Autodesk Inventor part; units mm, degrees
ref_plane "YZ Plane" through (0, 0, 0) normal (1, 0, 0) x (0, 1, 0)
ref_plane "XZ Plane" through (0, 0, 0) normal (0, 1, 0) x (-1, 0, 0)
ref_plane "XY Plane" through (0, 0, 0) normal (0, 0, 1) x (1, 0, 0)
sketch "Sketch1" plane through (0, 0, 0) normal (0, 0, 1) x (1, 0, 0)
  circle A0 centre (0, 0) radius 13.75
  circle A1 centre (0, 0) radius 18.75
  line L0 (-18.75, 0) -> (-38, 0)
  line L1 (-38, 0) -> (-38, -5)
  line L2 (-38, -5) -> (-18.75, -5)
  line L3 (-18.75, -5) -> (-18.75, 0)
  line L4 (-18.75, -5) -> (-13.75, -5)
  line L5 (-13.75, -5) -> (-13.75, 0)
  line L6 (-13.75, 0) -> (-18.75, 0)
  line L7 (-18.75, 0) -> (-18.75, -5)
  line L8 (18.75, 0) -> (38, 0)
  line L9 (38, 0) -> (38, -5)
  line L10 (38, -5) -> (18.75, -5)
  line L11 (18.75, -5) -> (18.75, 0)
  line L12 (18.75, -5) -> (13.75, -5)
  line L13 (13.75, -5) -> (13.75, 0)
  line L14 (13.75, 0) -> (18.75, 0)
  line L15 (18.75, 0) -> (18.75, -5)
  point P0 (-18.071, -5)
  point P1 (18.071, -5)
  dimension "d0" = 27.5
  dimension "d1" = 5
  dimension "d2" = 5
  dimension "d3" = 19.25
  dimension "d4" = 19.25
  dimension "d5" = 5
extrude "Extrusion1" add sketch "Sketch1" along normal blind 10 contours L13 L12 A1 L4 L5 A0 | L14 A1 L12 L13 | L5 L4 A1 L6 | L11 L12 A1 | L8 L9 L10 L11 | L3 L2 L1 L0 | A1 L4 L3
sketch "Sketch2" plane through (-38, -5, 0) normal (0, -1, 0) x (1, 0, 0)
  line L0 (0, 0) -> (19.929, 0)
  line L1 (19.929, 0) -> (19.929, 10)
  line L2 (0, 10) -> (19.929, 10)
  line L3 (0, 0) -> (0, 10)
  line L4 (56.071, 0) -> (76, 0)
  line L5 (76, 0) -> (76, 10)
  line L6 (56.071, 10) -> (76, 10)
  line L7 (56.071, 0) -> (56.071, 10)
  circle A0 centre (7.5, 5) radius 2.15
  circle A1 centre (68.5, 5) radius 2.15
  line L8 (0, 0) -> (0, 10)
  line L9 (76, 0) -> (76, 10)
  point P0 (38, 0)
  point P1 (9.9645, 10)
  point P2 (0, 5)
  point P3 (66.0355, 10)
  point P4 (76, 5)
  point P5 (0, 5)
  point P6 (0, 5)
  point P7 (76, 5)
  point P8 (76, 5)
  dimension "d8" = 4.3
  dimension "d9" = 4.3
  dimension "d13" = 7.5
  dimension "d14" = 7.5
extrude "Extrusion2" cut sketch "Sketch2" against normal up to surface (5 mm away) contours A0 | A1
fillet "Fillet1" radius 12 2 edges at (-18.071, -5, 5) (18.071, -5, 5)
equation "\"d4\" = d3"
Geometry: final body of the model. Coordinates: model frame, mm. A direction names the side the tool comes from. Give positions to 0.01 mm unless a question says otherwise; leave off trailing zeros. Write each loop counter-clockwise with the first axis right and the second up, starting at its lowest first coordinate (ties: lowest second). Pieces come first, ordered by that corner, then holes.
1. Section query D-D, the plane z = 2. Return loops of the section in (x, y), then the cut area to 3 significant figures.
2. Section query B-B, the plane z = 5. Return loops of the section in (x, y).
3. Section query C-C, the plane y = -9. Return loops of the section in (x, z), then the cut area to 3 significant figures.
4. Reachability of faces 1 (the flat face through (33, -5, 5)), 2 (the flat face through (-33, -5, 5)), 3 (the flat face through (-6, -13, 0)) from +Z, -Z, +X, -X, +Y, -Y: full face, straight path, thin tool, end or side. Return the list, or none.
5. Draft query along X for faces 4 (the flat face through (-26, 0, 5)), 5 (the cylindrical face through (-28.45, -2.54, 5.65)), 6 (the flat face through (38, -2, 5)). Return one class per face: released by +X, released by -X, zero draft, split by the parting line, or undercut.
6. Pin query (flat end, axial travel): P1, Ø4, axis at x = 30.5, z = 5, coming from the -Y side; P2, Ø5, axis at y = -16.5, z = 4, coming from the -X side; P3, Ø2, axis at x = 5, z = 2.5, coming from the -Y side; P4, Ø3, axis at x = -32.5, z = 4.5, coming from the -Y side. Return the tip coordinate at first contact, or that it passes through.
7. Line query: probe 1 along Z at (x, y) = (30.5, -3.2); probe 2 along X at (y, z) = (-7.5, 8.5); probe 3 along Y at (x, z) = (26, 2.25). Output: solid intervals per line, ascending.
8. Section query A-A, the plane x = 30.5. Return loops of the section in (y, z), then the cut area to 3 significant figures.
Computed:
1. outline: (-38, -5) - (-25.62, -5) arc R12 cw to (-15.62, -10.37) arc R18.75 ccw to (15.62, -10.37) arc R12 cw to (25.62, -5) - (38, -5) - (38, 0) - (13.75, 0) arc R13.75 cw to (-13.75, 0) - (-38, 0) - close
1. area: 467 mm2
2. outline: (-38, -5) - (-32.65, -5) - (-32.65, 0) - (-38, 0) - close; (-28.35, -5) - (-25.62, -5) arc R12 cw to (-15.62, -10.37) arc R18.75 ccw to (15.62, -10.37) arc R12 cw to (25.62, -5) - (28.35, -5) - (28.35, 0) - (13.75, 0) arc R13.75 cw to (-13.75, 0) - (-28.35, 0) - close; (32.65, -5) - (38, -5) - (38, 0) - (32.65, 0) - close
3. outline: (-16.68, 0) - (-10.4, 0) - (-10.4, 10) - (-16.68, 10) - close; (10.4, 0) - (16.68, 0) - (16.68, 10) - (10.4, 10) - close
3. area: 126 mm2
4. face 1: +Z, -Z, +X, -Y
4. face 2: +Z, -Z, -X, -Y
4. face 3: -Z, +X, -X, +Y, -Y
5. face 4: zero draft
5. face 5: undercut
5. face 6: released by +X
6. P1: passes through
6. P2: stops at x = -12.47
6. P3: stops at y = -18.32
6. P4: stops at y = -5
7. probe 1: z = 0 to 2.85, 7.15 to 10
7. probe 2: x = -18.29 to -11.52, 11.52 to 18.29
7. probe 3: y = -5 to 0
8. outline: (-5, 0) - (0, 0) - (0, 2.85) - (-5, 2.85) - close; (-5, 7.15) - (0, 7.15) - (0, 10) - (-5, 10) - close
8. area: 28.5 mm2
